Can you work these out from the model? Positions are in its coordinate system, mm. A direction names the side the tool comes from. Give positions to 0.01 mm unless a question says otherwise; leave off trailing zeros. Order: outer loops, then holes, each group sorted by start corner. A loop starts at its lowest first (then second) coordinate and runs counter-clockwise, first axis right, second up. Notation, with made-up numbers: M 38.5,8 L 74.5,8 A23 cw 74.5,29 Z; hole C -32.5,-26.5 d10. An arc over 180 degrees is marked long. One line per question, with ' | ' between items. Start each with the question number.
1) Please list where these lines run through material, in increasing order: line 1 along Y through (x, z) = (-5, 1.7); line 2 along Y through (x, z) = (0, 22.5); line 3 along X through (y, z) = (-5, 21). Write a range as [from, to].
2) If we section it at A-A, the plane z = 23: Please give me the cut outline in (x, y).
3) I'm going to push flat-ended pins straight in: pin 1 Ø12 at (x, y) = (-16.5, 23.5) entering from -Z; pin 2 Ø3.5 at (x, y) = (5, -25) entering from +Z; pin 3 Ø4 at (x, z) = (-24, -7.5) entering from -Y; pin 4 Ø20 at (y, z) = (15.5, 17.5) entering from +X. Where does each tip first touch, or does it pass through?
4) If we section it at D-D, the plane x = -19.5: Please give me the cut outline in (y, z), plus the area to 3 significant figures.
5) Thinking about a two-plate mould opening in X: for faces 1 (the flat face through (6.5, 53.5, 12.5)), 2 (the cylindrical face through (6.18, -13.92, 2.46)), 3 (the cylindrical face through (24, -9, 10)), 4 (the flat face through (-17, -22, 15)), which applies, +X half, -X half, draft (parallel to the pull), parting line (faces both ways), or undercut?
6) For faces 5 (the flat face through (25, -30, -13)), 6 (the flat face through (0, 40, 15)), 7 (the flat face through (22, -1, 12)), which set-ups out of +Z, -Z, +X, -X, +Y, -Y let a thin tool reach every point of the face, with its end or its side?
7) If we section it at C-C, the plane y = -25: Please give me the cut outline in (x, z), plus the area to 3 significant figures.
```python
from build123d import *

# Parameters (mm, degrees)
SKETCH_1_W          = 44
SKETCH_1_H          = 90
EXTRUDE_1_DEPTH     = 25
CUT_EXTRUDE_1_DEPTH = 20
SKETCH_3_W          = 5
SKETCH_3_H          = 20
EXTRUDE_2_DEPTH     = 20
FILLET_1_R          = 5
FILLET_START        = -22.5281
FILLET_3_DEPTH      = 0.5281
FILLET_START_2      = 22
FILLET_3_2_DEPTH    = 0.5137
FILLET_START_3      = 22.5137
FILLET_3_3_DEPTH    = 4.4863
FILLET_START_4      = -27
FILLET_3_4_DEPTH    = 4.4719
FILLET_START_5      = -20
FILLET_3_5_DEPTH    = 20
SKETCH_4_W          = 30
SKETCH_4_H          = 25
EXTRUDE_3_DEPTH     = 15
SKETCH_5_R          = 15
EXTRUDE_4_DEPTH     = 25
SKETCH_6_R          = 9
CUT_EXTRUDE_2_DEPTH = 25
FILLET_4_R          = 5
SKETCH_7_W          = 76.334334434
SKETCH_7_H          = 32
CUT_EXTRUDE_3_DEPTH = 20
SKETCH_9_W          = 10
SKETCH_9_H          = 40
CUT_EXTRUDE_5_DEPTH = 5
SKETCH_10_R         = 1.6
CUT_EXTRUDE_6_DEPTH = 5


with BuildPart() as part:
    # 草图1 → 凸台-拉伸1 (new body)
    with BuildSketch(Plane.XY):
        Rectangle(SKETCH_1_W, SKETCH_1_H)
    extrude(amount=EXTRUDE_1_DEPTH)

    # 草图2 → 切除-拉伸1 (cut)
    with BuildSketch(Plane.XY.offset(25)):
        Polygon((-17, 40), (17, 40), (17, -40), (17, -54.466657213), (-17, -54.466657213), (-17, -40), align=None)
    extrude(amount=-CUT_EXTRUDE_1_DEPTH, mode=Mode.SUBTRACT)

    # 草图3 → 凸台-拉伸2 (add, symmetric)
    with BuildSketch(Plane(origin=(0, 0, 0), x_dir=(-1, 0, 0), z_dir=(0, 0, -1))):
        with Locations((24.5, -20)):
            Rectangle(SKETCH_3_W, SKETCH_3_H)
        with Locations((-24.5, -20)):
            Rectangle(SKETCH_3_W, SKETCH_3_H)
    extrude(amount=EXTRUDE_2_DEPTH, both=True)

    # 圆角1
    fillet_1_edges = [part.edges().sort_by_distance(p)[0] for p in [
        (22, -30, 10),
        (-22, -30, 10),
        (-22, -10, 10),
        (22, -10, 10),
    ]]
    fillet(fillet_1_edges, radius=FILLET_1_R - 0.0001)  # a hair under: the kernel refuses the full size

    # 圆角3: read off the stored shape, not the designer's step
    # 圆角3 outline → 圆角3 (add)
    with BuildSketch(Plane.YZ.offset(FILLET_START)):
        with BuildLine():
            Line((-5, 0), (-10, 0))
            Line((-10, 0), (-10, -5))
            ThreePointArc((-10, -5), (-8.535533906, -1.464466094), (-5, 0))
        make_face()
        with BuildLine():
            ThreePointArc((-35, 0), (-31.464466094, -1.464466094), (-30, -5))
            Line((-30, -5), (-30, 0))
            Line((-30, 0), (-35, 0))
        make_face()
    extrude(amount=FILLET_3_DEPTH)

    # Fillet 3 2 outline → Fillet 3 2 (add)
    with BuildSketch(Plane.YZ.offset(FILLET_START_2)):
        with BuildLine():
            Line((-5, 0), (-10, 0))
            Line((-10, 0), (-10, -5))
            ThreePointArc((-10, -5), (-8.535533906, -1.464466094), (-5, 0))
        make_face()
        with BuildLine():
            ThreePointArc((-35, 0), (-31.464466094, -1.464466094), (-30, -5))
            Line((-30, -5), (-30, 0))
            Line((-30, 0), (-35, 0))
        make_face()
    extrude(amount=FILLET_3_2_DEPTH)

    # Fillet 3 3 outline → Fillet 3 3 (add)
    with BuildSketch(Plane.YZ.offset(FILLET_START_3)):
        with BuildLine():
            ThreePointArc((-35, 0), (-31.464466094, -1.464466094), (-30, -5))
            Line((-30, -5), (-30, 0))
            Line((-30, 0), (-35, 0))
        make_face()
        with BuildLine():
            Line((-10, 0), (-10, -5))
            ThreePointArc((-10, -5), (-8.535533906, -1.464466094), (-5, 0))
            Line((-5, 0), (-10, 0))
        make_face()
    extrude(amount=FILLET_3_3_DEPTH)

    # Fillet 3 4 outline → Fillet 3 4 (add)
    with BuildSketch(Plane.YZ.offset(FILLET_START_4)):
        with BuildLine():
            ThreePointArc((-35, 0), (-31.464466094, -1.464466094), (-30, -5))
            Line((-30, -5), (-30, 0))
            Line((-30, 0), (-35, 0))
        make_face()
        with BuildLine():
            Line((-10, 0), (-10, -5))
            ThreePointArc((-10, -5), (-8.535533906, -1.464466094), (-5, 0))
            Line((-5, 0), (-10, 0))
        make_face()
    extrude(amount=FILLET_3_4_DEPTH)

    # Fillet 3 5 outline → Fillet 3 5 (cut)
    with BuildSketch(Plane.XY.offset(FILLET_START_5)):
        with BuildLine():
            ThreePointArc((27, -30), (23.464466094, -31.464466094), (22, -35))
            Line((22, -35), (22, -36))
            Line((22, -36), (27, -36))
            Line((27, -36), (27, -30))
        make_face()
        with BuildLine():
            ThreePointArc((22, -5), (23.464466094, -8.535533906), (27, -10))
            Line((27, -10), (27, -3))
            Line((27, -3), (22, -3))
            Line((22, -3), (22, -5))
        make_face()
        with BuildLine():
            Line((-27, -36), (-22, -36))
            Line((-22, -36), (-22, -35))
            ThreePointArc((-22, -35), (-23.464466094, -31.464466094), (-27, -30))
            Line((-27, -30), (-27, -36))
        make_face()
        with BuildLine():
            Line((-22, -5), (-22, -3))
            Line((-22, -3), (-27, -3))
            Line((-27, -3), (-27, -10))
            ThreePointArc((-27, -10), (-23.464466094, -8.535533906), (-22, -5))
        make_face()
    extrude(amount=FILLET_3_5_DEPTH, mode=Mode.SUBTRACT)

    # 草图4 → 凸台-拉伸3 (add)
    with BuildSketch(Plane(origin=(0, 45, 0), x_dir=(1, 0, 0), z_dir=(0, 1, 0))):
        with Locations((0, -25)):
            Rectangle(SKETCH_4_W, SKETCH_4_H)
    extrude(amount=EXTRUDE_3_DEPTH)

    # 草图5 → 凸台-拉伸4 (add)
    with BuildSketch(Plane.XY.offset(37.5)):
        with Locations((0, 60)):
            Circle(SKETCH_5_R)
    extrude(amount=-EXTRUDE_4_DEPTH)

    # 草图6 → 切除-拉伸2 (cut)
    with BuildSketch(Plane.XY.offset(37.5)):
        with Locations((0, 60)):
            Circle(SKETCH_6_R)
    extrude(amount=-CUT_EXTRUDE_2_DEPTH, mode=Mode.SUBTRACT)

    # 圆角4
    fillet_4_edges = [part.edges().sort_by_distance(p)[0] for p in [
        (0, 45, 25),
    ]]
    fillet(fillet_4_edges, radius=FILLET_4_R - 0.0001)  # a hair under: the kernel refuses the full size

    # 草图7 → 切除-拉伸3 (cut)
    with BuildSketch(Plane.XY.offset(25)):
        with Locations((0, 16)):
            Rectangle(SKETCH_7_W, SKETCH_7_H)
    extrude(amount=-CUT_EXTRUDE_3_DEPTH, mode=Mode.SUBTRACT)

    # 草图9 → 切除-拉伸5 (cut)
    with BuildSketch(Plane(origin=(0, 0, -20), x_dir=(-1, 0, 0), z_dir=(0, 0, -1))):
        with Locations((22, -10)):
            Rectangle(SKETCH_9_W, SKETCH_9_H)
    extrude(amount=-CUT_EXTRUDE_5_DEPTH, mode=Mode.SUBTRACT)

    # 草图10 → 切除-拉伸6 (cut)
    with BuildSketch(Plane(origin=(0, 0, 0), x_dir=(-1, 0, 0), z_dir=(0, 0, -1))):
        with Locations((5, -15)):
            Circle(SKETCH_10_R)
        with Locations((5, -25)):
            Circle(SKETCH_10_R)
        with Locations((-5, -25)):
            Circle(SKETCH_10_R)
        with Locations((-5, -15)):
            Circle(SKETCH_10_R)
    extrude(amount=-CUT_EXTRUDE_6_DEPTH, mode=Mode.SUBTRACT)


solid = part.part
```
Results found:
1) line 1: y = [-45, -26.6], [-23.4, -16.6], [-13.4, 45] | line 2: y = [40, 51], [69, 75] | line 3: x = [-22, -17], [17, 22]
2) outline: M -22,-45 L -17,-45 L -17,0 L -22,0 Z; M -22,32 L -17,32 L -17,40 L 17,40 L 17,32 L 22,32 L 22,45 L 15,45 L 15,60 A15 ccw -15,60 L -15,45 L -22,45 Z; M 17,-45 L 22,-45 L 22,0 L 17,0 Z; hole C 0,60 d18
3) pin 1: stops at z = 0 | pin 2: stops at z = 5 | pin 3: stops at y = -30 | pin 4: passes through
4) outline: M -45,0 L 45,0 L 45,25 L 32,25 L 32,5 L 0,5 L 0,25 L -45,25 Z | area: 1,610 mm²
5) face 1: draft | face 2: undercut | face 3: +X half | face 4: undercut
6) face 5: -Z, +X, -X, -Y | face 6: +Z, -Y | face 7: +Z, +X
7) outline: M -27,-15 L -22,-15 L -22,0 L -6.6,0 L -6.6,5 L -17,5 L -17,25 L -22,25 L -22,20 L -27,20 Z; M -3.4,0 L 3.4,0 L 3.4,5 L -3.4,5 Z; M 6.6,0 L 22,0 L 22,-20 L 27,-20 L 27,20 L 22,20 L 22,25 L 17,25 L 17,5 L 6.6,5 Z | area: 763 mm²
